The listing builds one solid part. Answer for the finished solid, in the listing's coordinates (mm). Face numbers are marked on the shaded views. Round coordinates to 2 decimals unless told otherwise and drop trailing zeros. Write each loop counter-clockwise with the first axis right and the second up, starting at its lowest first coordinate (ties: lowest second). Pieces come first, ordered by that corner, then holes.
(1) A cutting plane is placed at D-D, the plane x = 27.5. Give the vertices of the cut face in (y, z).
(2) Each of these flat-tipped pins is pushed along its axis until it touches: pin 1 Ø19 at (x, z) = (-10, -15) entering from +Y; pin 2 Ø2 at (x, y) = (-11, -2) entering from -Z; pin 3 Ø4 at (x, z) = (42.6, 24.6) entering from +Y; pin 4 Ø0.8 at (x, y) = (-15.5, -5) entering from -Z. Where does it stop, or does it pass through?
(3) The mould has two halves that part along X. Classify the marked faces 1 and 2: +X half, -X half, draft (parallel to the pull), parting line (faces both ways), or undercut.
(4) A cutting plane is placed at C-C, the plane z = -26.3. Give the vertices of the cut face in (x, y).
(5) A cutting plane is placed at A-A, the plane x = -41.4. Give the vertices of the cut face in (y, z).
(6) Find the intervals of material crossed by probe 1 along X at (y, z) = (-2, 24.6); probe 2 along Z at (x, y) = (42.6, -1.5); probe 3 along X at (y, z) = (-4.75, -26.3), in increasing order.
(7) A cutting plane is placed at B-B, the plane y = -2.5. Give the vertices of the cut face in (x, z), and give its area (3 significant figures).
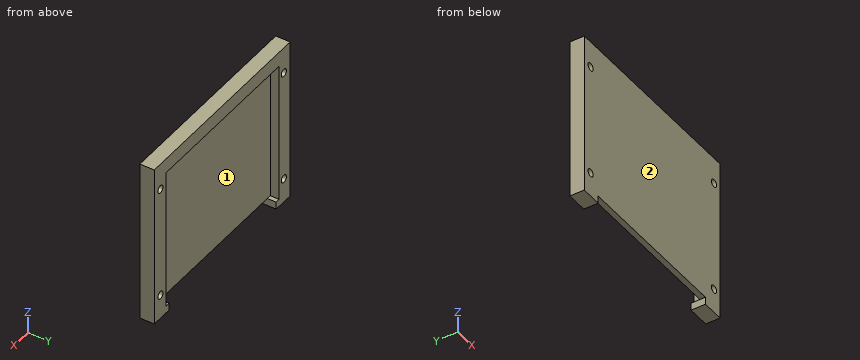
from build123d import *

# Parameters (mm, degrees)
F0_W     = 71.45
F0_H     = 53.85
F1_DEPTH = 6.5
F0_W_2   = 73
F0_H_2   = 3.35
F2_DEPTH = 4
F3_D     = 3.5


with BuildPart() as f1:
    # F0 (on Front) → F1 (new body)
    with BuildSketch(Plane.XZ):
        Polygon((-38.2, -34.05), (-38.2, 29.95), (38.8, 29.95), (38.8, -34.05), (36.8, -34.05), (36.8, -37.4), (46.8, -37.4), (46.8, 36.6), (-45.7, 36.6), (-45.7, -37.4), (-36.2, -37.4), (-36.2, -34.05), align=None)
        Polygon((38.8, 29.95), (-38.2, 29.95), (-38.2, -34.05), (-36.2, -34.05), (36.8, -34.05), (38.8, -34.05), align=None)
        with Locations((-0.025, -0.025)):
            Rectangle(F0_W, F0_H, mode=Mode.SUBTRACT)
        with Locations((-0.025, -0.025)):
            Rectangle(F0_W, F0_H)
    extrude(amount=F1_DEPTH)

    # F0 (on Front) → F2 (cut)
    with BuildSketch(Plane.XZ):
        Polygon((38.8, 29.95), (-38.2, 29.95), (-38.2, -34.05), (-36.2, -34.05), (36.8, -34.05), (38.8, -34.05), align=None)
        with Locations((-0.025, -0.025)):
            Rectangle(F0_W, F0_H, mode=Mode.SUBTRACT)
        with Locations((-0.025, -0.025)):
            Rectangle(F0_W, F0_H)
        with Locations((0.3, -35.725)):
            Rectangle(F0_W_2, F0_H_2)
    extrude(amount=F2_DEPTH, mode=Mode.SUBTRACT)

    # F3 (through all)
    with Locations(Plane(origin=(0, 0, 0), x_dir=(1, 0, 0), z_dir=(0, 1, 0))):
        with Locations((-41.4, -24.6), (42.6, -24.6), (42.6, 26.3), (-41.4, 26.3)):
            Hole(F3_D / 2)


solid = f1.part
Solutions:
1. outline: (-6.5, -34.05) - (-4, -34.05) - (-4, 29.95) - (0, 29.95) - (0, 36.6) - (-6.5, 36.6) - close
2. pin 1: stops at y = -4
2. pin 2: stops at z = 29.95
2. pin 3: stops at y = 0
2. pin 4: stops at z = -34.05
3. face 1: undercut
3. face 2: draft
4. outline: (-45.7, -6.5) - (-43.15, -6.5) - (-43.15, 0) - (-45.7, 0) - close; (-39.65, -6.5) - (40.85, -6.5) - (40.85, 0) - (38.8, 0) - (38.8, -4) - (-38.2, -4) - (-38.2, 0) - (-39.65, 0) - close; (44.35, -6.5) - (46.8, -6.5) - (46.8, 0) - (44.35, 0) - close
5. outline: (-6.5, -37.4) - (0, -37.4) - (0, -28.05) - (-6.5, -28.05) - close; (-6.5, -24.55) - (0, -24.55) - (0, 22.85) - (-6.5, 22.85) - close; (-6.5, 26.35) - (0, 26.35) - (0, 36.6) - (-6.5, 36.6) - close
6. probe 1: x = -45.7 to -43.15, -39.65 to -38.2, 38.8 to 40.85, 44.35 to 46.8
6. probe 2: z = -37.4 to -28.05, -24.55 to 22.85, 26.35 to 36.6
6. probe 3: x = -45.7 to -43.15, -39.65 to 40.85, 44.35 to 46.8
7. outline: (-45.7, -37.4) - (-36.2, -37.4) - (-36.2, -34.05) - (-38.2, -34.05) - (-38.2, 29.95) - (38.8, 29.95) - (38.8, -34.05) - (36.8, -34.05) - (36.8, -37.4) - (46.8, -37.4) - (46.8, 36.6) - (-45.7, 36.6) - close; hole circle Ø3.5 at (-41.4, -26.3); hole circle Ø3.5 at (-41.4, 24.6); hole circle Ø3.5 at (42.6, -26.3); hole circle Ø3.5 at (42.6, 24.6)
7. area: 1,630 mm2
